Work out the finished part from the listing and answer in its coordinate system (mm). A direction names the side the tool comes from. Coordinates: 2 decimals unless noted, no trailing zeros. Order: outer loops, then holes, each group sorted by start corner. A loop starts at its lowest first (then second) coordinate and runs counter-clockwise, first axis right, second up. Notation, with made-up numbers: M 46,47.5 L 99,47.5 A11 ccw 99,66.5 Z; hole C 6,-24.75 d8. An arc over 180 degrees is marked long. Use a Markdown table: item, result.
from build123d import *

# Parameters (mm, degrees)
BOSS_EXTRUDE1_DEPTH   = 2
F_1_CLEARANCE_HOLE1_D = 2.20000068
FILLET1_R             = 0.8


with BuildPart() as part:
    # Sketch1 → Boss-Extrude1 (new body)
    with BuildSketch(Plane(origin=(0, 0, -2), x_dir=(-1, 0, 0), z_dir=(0, 0, -1))):
        with BuildLine():
            Line((-1.91693771, 8.900326187), (-9.84300771, 8.900326187))
            Line((-9.84300771, 8.900326187), (-9.84300771, 1.196506187))
            ThreePointArc((-9.84300771, 1.196506187), (-11.94993771, -0.910423813), (-9.84300771, -3.017353813))
            Line((-9.84300771, -3.017353813), (-9.84300771, -10.943423813))
            Line((-9.84300771, -10.943423813), (-1.91693771, -10.943423813))
            ThreePointArc((-1.91693771, -10.943423813), (0.18999229, -13.050353813), (2.29692229, -10.943423813))
            Line((2.29692229, -10.943423813), (10.00074229, -10.943423813))
            Line((10.00074229, -10.943423813), (10.00074229, -3.017353813))
            ThreePointArc((10.00074229, -3.017353813), (12.10767229, -0.910423813), (10.00074229, 1.196506187))
            Line((10.00074229, 1.196506187), (10.00074229, 8.900326187))
            Line((10.00074229, 8.900326187), (2.29692229, 8.900326187))
            ThreePointArc((2.29692229, 8.900326187), (0.18999229, 11.007256187), (-1.91693771, 8.900326187))
        make_face()
    extrude(amount=-BOSS_EXTRUDE1_DEPTH)

    # #1 Clearance Hole1 (through all)
    with Locations(Plane(origin=(0, 0, -2), x_dir=(-1, 0, 0), z_dir=(0, 0, -1))):
        with Locations((0.189367378, -10.907429297), (0.189367378, 9.092570703), (10.189367378, -0.907429297), (-9.810632622, -0.907429297)):
            Hole(F_1_CLEARANCE_HOLE1_D / 2)

    # Fillet1
    fillet1_edges = [part.edges().sort_by_distance(p)[0] for p in [
        (-10.00074229, 8.900326187, -1),
        (-10.00074229, -10.943423813, -1),
        (9.84300771, -10.943423813, -1),
        (9.84300771, 8.900326187, -1),
    ]]
    fillet(fillet1_edges, radius=FILLET1_R)


solid = part.part
(1) Determine the mould class of faces 1 (the cylindrical face through (-0.333, 10.183, -0.986)), 2 (the cylindrical face through (10.86, -0.58, -0.99)), 3 (the flat face through (5, 8.9, -1)), 4 (the flat face through (9.843, 5, -1)) for opening direction X: pulls with the +X half, pulls with the -X half, needs draft (parallel to the pull), parting line crosses it, or undercut.
Conclusion:
| item | result |
|---|---|
| face 1 | undercut |
| face 2 | undercut |
| face 3 | needs draft |
| face 4 | pulls with the +X half |
(2) A cutting plane is placed at B-B (x = 0.25). Determine the outline of the cut face in (y, z), then the cut area to 3 significant figures.
Conclusion:
| item | result |
|---|---|
| outline | M -13,-2 L -11.92,-2 L -11.92,0 L -13,0 Z; M -9.9,-2 L 8.08,-2 L 8.08,0 L -9.9,0 Z; M 10.1,-2 L 10.96,-2 L 10.96,0 L 10.1,0 Z |
| area | 39.9 mm2 |
(3) Given P1, Ø0.6, axis at x = -6, z = -1, coming from the +Y side; P2, Ø0.6, axis at y = -7.5, z = -1, coming from the -X side; P3, Ø1, axis at y = -5.5, z = -0.5, coming from the +X side, each flat-ended and moving along its own axis, determine where each tip first touches the part or whether it passes through.
Conclusion:
| item | result |
|---|---|
| P1 | y = 8.9 |
| P2 | x = -10 |
| P3 | x = 9.84 |
(4) A cutting plane is placed at C-C (y = -1.5). Determine the outline of the cut face in (x, z).
Conclusion:
| item | result |
|---|---|
| outline | M -12.02,-2 L -11.12,-2 L -11.12,0 L -12.02,0 Z; M -9.26,-2 L 8.88,-2 L 8.88,0 L -9.26,0 Z; M 10.74,-2 L 11.87,-2 L 11.87,0 L 10.74,0 Z |
(5) A cutting plane is placed at D-D (x = 5.5). Determine the outline of the cut face in (y, z).
Conclusion:
| item | result |
|---|---|
| outline | M -10.94,-2 L 8.9,-2 L 8.9,0 L -10.94,0 Z |
(6) A cutting plane is placed at A-A (z = -0.9). Determine the outline of the cut face in (x, y).
Conclusion:
| item | result |
|---|---|
| outline | M -10,-10.14 A0.8 ccw -9.2,-10.94 L -2.3,-10.94 A2.11 ccw 1.92,-10.94 L 9.04,-10.94 A0.8 ccw 9.84,-10.14 L 9.84,-3.02 A2.11 ccw 9.84,1.2 L 9.84,8.1 A0.8 ccw 9.04,8.9 L 1.92,8.9 A2.11 ccw -2.3,8.9 L -9.2,8.9 A0.8 ccw -10,8.1 L -10,1.2 A2.11 ccw -10,-3.02 Z; hole C -10.19,-0.91 d2.2; hole C -0.19,-10.91 d2.2; hole C -0.19,9.09 d2.2; hole C 9.81,-0.91 d2.2 |
(7) Which of the six approach directions +Z, -Z, +X, -X, +Y, -Y give full straight-line access (tool end or side, diameter ignored) to faces 5 (the flat face through (6, -10.943, -1)), 6 (the cylindrical face through (0, 11, -1)), 7 (the flat face through (-6, 8.9, -1))?
Conclusion:
| item | result |
|---|---|
| face 5 | +Z, -Z, +X, -Y |
| face 6 | +Z, -Z, +Y |
| face 7 | +Z, -Z, -X, +Y |
(8) Straight lines are drawn through the part: L1, parallel to X at y = -11, z = -0.2; L2, parallel to Y at x = -0.5, z = -1.85; L3, parallel to X at y = 0, z = -0.15. For each, find the intervals that lie inside material, in ascending order.
Conclusion:
| item | result |
|---|---|
| L1 | -2.3 to -1.29, 0.91 to 1.92 |
| L2 | -13.03 to -11.96, -9.85 to 8.04, 10.15 to 10.98 |
| L3 | -11.9 to -10.81, -9.57 to 9.19, 10.43 to 11.74 |
